Check sheet for the drawn part. Datum: minimum x, y, z corner. Units: mm. Coordinates: 2 decimals unless noted, no trailing zeros. Loops run counter-clockwise (first coordinate to the right, second up) from the corner with the lowest first, then second, coordinate; pieces in that order, holes last.
Q1. Sectioned sample at D-D (z = 3.9). Enter the section's corners in (x, y).
Q2. Mould release check, pull along Y, two halves, no side actions. Record for the marked faces 1, 2 and 3: +Y half, -Y half, draft (parallel to the pull), parting line (faces both ways), or undercut.
Q3. Sectioned sample at C-C (y = 6.5). Enter the section's corners in (x, z), then the cut area to 3 significant figures.
Q4. Sectioned sample at A-A (y = 20). Enter the section's corners in (x, z), then the cut area to 3 significant figures.
Q5. Go/stop test with flat-tipped pins: P1, Ø2, axis at x = 4.5, z = 1, coming from the +Y side (3 decimals); P2, Ø1.5, axis at y = 33, z = 4, coming from the -X side. Record where each tip stops, or that it passes through.
Q6. Material ranges on probe 1 along Y at (x, z) = (20, 2.15); probe 2 along Y at (x, z) = (20.5, 4.45), recorded low to high.
Q7. Sectioned sample at B-B (x = 35.5). Enter the section's corners in (y, z), then the cut area to 3 significant figures.
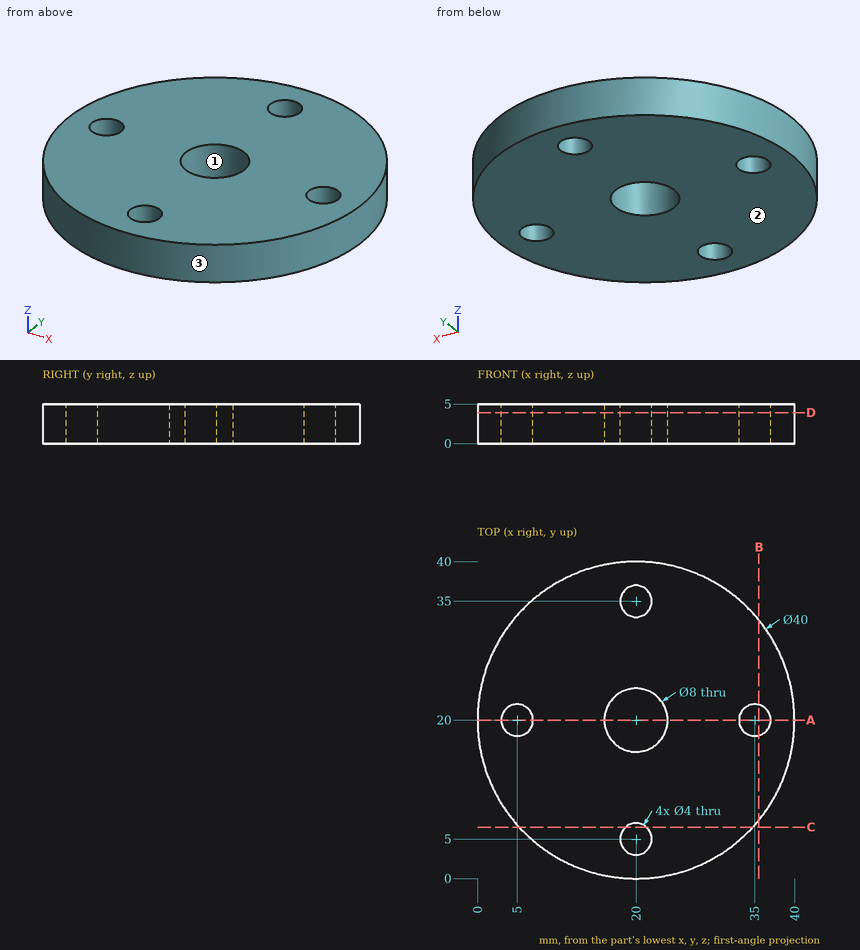
Geometry check:
1. outline: circle Ø40 at (20, 20); hole circle Ø4 at (5, 20); hole circle Ø8 at (20, 20); hole circle Ø4 at (20, 5); hole circle Ø4 at (20, 35); hole circle Ø4 at (35, 20)
2. face 1: undercut
2. face 2: draft
2. face 3: parting line
3. outline: (5.24, 0) - (18.68, 0) - (18.68, 5) - (5.24, 5) - close; (21.32, 0) - (34.76, 0) - (34.76, 5) - (21.32, 5) - close
3. area: 134 mm2
4. outline: (0, 0) - (3, 0) - (3, 5) - (0, 5) - close; (7, 0) - (16, 0) - (16, 5) - (7, 5) - close; (24, 0) - (33, 0) - (33, 5) - (24, 5) - close; (37, 0) - (40, 0) - (40, 5) - (37, 5) - close
4. area: 120 mm2
5. P1: stops at y = 33.775
5. P2: stops at x = 4.19
6. probe 1: y = 0 to 3, 7 to 16, 24 to 33, 37 to 40
6. probe 2: y = 0.01 to 3.06, 6.94 to 16.03, 23.97 to 33.06, 36.94 to 39.99
7. outline: (7.36, 0) - (18.06, 0) - (18.06, 5) - (7.36, 5) - close; (21.94, 0) - (32.64, 0) - (32.64, 5) - (21.94, 5) - close
7. area: 107 mm2
